Check sheet for the modelled part. Datum: model origin and axes. Units: mm. Give positions to 0.01 mm unless a question says otherwise; leave off trailing zeros. Order: outer loops, then holes, each group sorted by start corner. A loop starts at its lowest first (then second) coordinate and runs counter-clockwise, first axis right, second up.
```python
from build123d import *

# Parameters (mm, degrees)
SKETCH_1_W           = 180
SKETCH_1_H           = 180
EXTRUDE_1_DEPTH      = 3
CUT_EXTRUDE_1_DEPTH  = 3
SKETCH_3_R           = 2.1
CUT_EXTRUDE_2_DEPTH  = 3
SKETCH_4_R           = 25
SKETCH_4_R_2         = 1.5
CUT_EXTRUDE_3_DEPTH  = 3
SKETCH_5_R           = 1.5
SKETCH_5_R_2         = 5
CUT_EXTRUDE_4_DEPTH  = 3
SKETCH_6_R           = 1.5
CUT_EXTRUDE_5_DEPTH  = 3
FILLET_2_R           = 5
SKETCH_7_R           = 1.5
CUT_EXTRUDE_6_DEPTH  = 3
SKETCH_8_R           = 1.5
CUT_EXTRUDE_7_DEPTH  = 3
SKETCH_10_R          = 1.5
CUT_EXTRUDE_9_DEPTH  = 3
SKETCH_11_R          = 1.5
SKETCH_11_R_2        = 4
CUT_EXTRUDE_10_DEPTH = 3
SKETCH_12_R          = 3
CUT_EXTRUDE_11_DEPTH = 3
SKETCH_13_R          = 1.75
CUT_EXTRUDE_12_DEPTH = 3


with BuildPart() as part:
    # 草图1 → 凸台-拉伸1 (new body)
    with BuildSketch(Plane.XY):
        Rectangle(SKETCH_1_W, SKETCH_1_H)
    extrude(amount=EXTRUDE_1_DEPTH)

    # 草图2 → 切除-拉伸1 (cut)
    with BuildSketch(Plane.XY.offset(3)):
        Polygon((-90, 90), (-55, 90), (-90, 55), align=None)
        Polygon((90, 90), (55, 90), (90, 55), align=None)
        Polygon((-90, -90), (-90, -55), (-55, -90), align=None)
        Polygon((90, -90), (90, -55), (55, -90), align=None)
    extrude(amount=-CUT_EXTRUDE_1_DEPTH, mode=Mode.SUBTRACT)

    # 草图3 → 切除-拉伸2 (cut)
    with BuildSketch(Plane.XY.offset(3)):
        with Locations((55.529437252, 76.742640687)):
            Circle(SKETCH_3_R)
        with Locations((76.742640687, 55.529437252)):
            Circle(SKETCH_3_R)
        with Locations((59.064971157, 37.851767722)):
            Circle(SKETCH_3_R)
        with Locations((37.851767722, 59.064971157)):
            Circle(SKETCH_3_R)
        with Locations((-55.529437252, 76.742640687)):
            Circle(SKETCH_3_R)
        with Locations((-37.851767722, 59.064971157)):
            Circle(SKETCH_3_R)
        with Locations((-59.064971157, 37.851767722)):
            Circle(SKETCH_3_R)
        with Locations((-76.742640687, 55.529437252)):
            Circle(SKETCH_3_R)
        with Locations((-59.064971157, -37.851767722)):
            Circle(SKETCH_3_R)
        with Locations((-76.742640687, -55.529437252)):
            Circle(SKETCH_3_R)
        with Locations((-37.851767722, -59.064971157)):
            Circle(SKETCH_3_R)
        with Locations((-55.529437252, -76.742640687)):
            Circle(SKETCH_3_R)
        with Locations((76.742640687, -55.529437252)):
            Circle(SKETCH_3_R)
        with Locations((55.529437252, -76.742640687)):
            Circle(SKETCH_3_R)
        with Locations((37.851767722, -59.064971157)):
            Circle(SKETCH_3_R)
        with Locations((59.064971157, -37.851767722)):
            Circle(SKETCH_3_R)
    extrude(amount=-CUT_EXTRUDE_2_DEPTH, mode=Mode.SUBTRACT)

    # 草图4 → 切除-拉伸3 (cut)
    with BuildSketch(Plane.XY.offset(3)):
        Circle(SKETCH_4_R)
        with Locations((67.5, 26)):
            Circle(SKETCH_4_R_2)
        with Locations((67.5, -26)):
            Circle(SKETCH_4_R_2)
        with Locations((-67.5, -26)):
            Circle(SKETCH_4_R_2)
        with Locations((-67.5, 26)):
            Circle(SKETCH_4_R_2)
    extrude(amount=-CUT_EXTRUDE_3_DEPTH, mode=Mode.SUBTRACT)

    # 草图5 → 切除-拉伸4 (cut)
    with BuildSketch(Plane.XY.offset(3)):
        with Locations((61, 9.75)):
            Circle(SKETCH_5_R)
        with Locations((61, -9.75)):
            Circle(SKETCH_5_R)
        with Locations((80, 0)):
            Circle(SKETCH_5_R_2)
        with Locations((35, 22.5)):
            Circle(SKETCH_5_R)
        with Locations((35, -22.5)):
            Circle(SKETCH_5_R)
        with Locations((80, -22.5)):
            Circle(SKETCH_5_R)
        with Locations((80, 22.5)):
            Circle(SKETCH_5_R)
        with Locations((-80, 22.5)):
            Circle(SKETCH_5_R)
        with Locations((-80, -22.5)):
            Circle(SKETCH_5_R)
        with Locations((-35, -22.5)):
            Circle(SKETCH_5_R)
        with Locations((-35, 22.5)):
            Circle(SKETCH_5_R)
        with Locations((-61, 9.75)):
            Circle(SKETCH_5_R)
        with Locations((-61, -9.75)):
            Circle(SKETCH_5_R)
        with Locations((-80, 0)):
            Circle(SKETCH_5_R_2)
    extrude(amount=-CUT_EXTRUDE_4_DEPTH, mode=Mode.SUBTRACT)

    # 草图6 → 切除-拉伸5 (cut)
    with BuildSketch(Plane.XY.offset(3)):
        with Locations((14.820508076, 25.669872981)):
            Circle(SKETCH_6_R)
        with Locations((-14.820508076, 25.669872981)):
            Circle(SKETCH_6_R)
        with Locations((-30, 0)):
            Circle(SKETCH_6_R)
        with Locations((-14.820508076, -25.669872981)):
            Circle(SKETCH_6_R)
        with Locations((14.820508076, -25.669872981)):
            Circle(SKETCH_6_R)
        with Locations((30, 0)):
            Circle(SKETCH_6_R)
    extrude(amount=-CUT_EXTRUDE_5_DEPTH, mode=Mode.SUBTRACT)

    # 圆角2
    fillet_2_edges = [part.edges().sort_by_distance(p)[0] for p in [
        (90, 55, 1.5),
        (55, 90, 1.5),
        (-55, -90, 1.5),
        (-90, -55, 1.5),
        (55, -90, 1.5),
        (90, -55, 1.5),
        (-90, 55, 1.5),
        (-55, 90, 1.5),
    ]]
    fillet(fillet_2_edges, radius=FILLET_2_R)

    # 草图7 → 切除-拉伸6 (cut)
    with BuildSketch(Plane.XY.offset(3)):
        with Locations((-25, 65.6)):
            Circle(SKETCH_7_R)
        with Locations((25, 65.6)):
            Circle(SKETCH_7_R)
    extrude(amount=-CUT_EXTRUDE_6_DEPTH, mode=Mode.SUBTRACT)

    # 草图8 → 切除-拉伸7 (cut)
    with BuildSketch(Plane.XY.offset(3)):
        with Locations((25, -65.6)):
            Circle(SKETCH_8_R)
        with Locations((-25, -65.6)):
            Circle(SKETCH_8_R)
    extrude(amount=-CUT_EXTRUDE_7_DEPTH, mode=Mode.SUBTRACT)

    # 草图10 → 切除-拉伸9 (cut)
    with BuildSketch(Plane.XY.offset(3)):
        with Locations((-47, -84)):
            Circle(SKETCH_10_R)
        with Locations((47, -84)):
            Circle(SKETCH_10_R)
        with Locations((-84, -45)):
            Circle(SKETCH_10_R)
        with Locations((-84, 45)):
            Circle(SKETCH_10_R)
        with Locations((84, -45)):
            Circle(SKETCH_10_R)
        with Locations((84, 45)):
            Circle(SKETCH_10_R)
        with Locations((-45, 84)):
            Circle(SKETCH_10_R)
        with Locations((45, 84)):
            Circle(SKETCH_10_R)
    extrude(amount=-CUT_EXTRUDE_9_DEPTH, mode=Mode.SUBTRACT)

    # 草图11 → 切除-拉伸10 (cut)
    with BuildSketch(Plane.XY.offset(3)):
        with Locations((9.75, -57.5)):
            Circle(SKETCH_11_R)
        with Locations((-9.75, -57.5)):
            Circle(SKETCH_11_R)
        with Locations((0, -83)):
            Circle(SKETCH_11_R_2)
    extrude(amount=-CUT_EXTRUDE_10_DEPTH, mode=Mode.SUBTRACT)

    # 草图12 → 切除-拉伸11 (cut)
    with BuildSketch(Plane.XY.offset(3)):
        with Locations((0, 69.9)):
            Circle(SKETCH_12_R)
    extrude(amount=-CUT_EXTRUDE_11_DEPTH, mode=Mode.SUBTRACT)

    # 草图13 → 切除-拉伸12 (cut)
    with BuildSketch(Plane.XY.offset(3)):
        with Locations((-13.5, 79.940916293)):
            Circle(SKETCH_13_R)
        with Locations((-13.5, 59.859083707)):
            Circle(SKETCH_13_R)
        with Locations((13.5, 59.859083707)):
            Circle(SKETCH_13_R)
        with Locations((13.5, 79.940916293)):
            Circle(SKETCH_13_R)
    extrude(amount=-CUT_EXTRUDE_12_DEPTH, mode=Mode.SUBTRACT)


solid = part.part
```
(1) Release check for a two-part mould opening along X. For faces 1 (the face through (72, 73, 2)), 2 (the face through (-21, 21, 3)), 3 (the face through (61.07, 38.48, 1.52)) record: released by +X, released by -X, zero draft, split by the parting line, or undercut.
(2) Thickness scan on L1, parallel to X at y = -66, z = 0.3; L2, parallel to X at y = 65.6, z = 0.6; L3, parallel to Y at x = -61, z = 0.9. Record the ranges inside material, lowest first.
(3) Go/stop test with a flat-tipped pin: P1, Ø1.5, axis at x = -67, z = 2, coming from the +Y side. Record where the tip stops, or that it passes through.
(4) Sectioned sample at B-B (z = 1.4). Count the separate pieces of the cut face and the enclosed holes in it, plus the area to 3 significant figures.
(5) Sectioned sample at A-A (y = 15). Enter the section's corners in (x, z), plus the area to 3 significant figures.
Values follow:
1. face 1: released by +X
1. face 2: zero draft
1. face 3: undercut
2. L1: x = -79 to -26.45, -23.55 to 23.55, 26.45 to 79
2. L2: x = -79.4 to -26.5, -23.5 to 23.5, 26.5 to 79.4
2. L3: y = -84 to -38.67, -37.04 to -11.25, -8.25 to 8.25, 11.25 to 37.04, 38.67 to 84
3. P1: stops at y = 78.75
4. separate pieces: 1
4. enclosed holes: 61
4. area: 27,200 mm2
5. outline: (-90, 0) - (-20, 0) - (-20, 3) - (-90, 3) - close; (20, 0) - (90, 0) - (90, 3) - (20, 3) - close
5. area: 420 mm2
